Check sheet for the modelled part. Datum: model origin and axes. Units: mm. Round coordinates to 2 decimals unless told otherwise and drop trailing zeros. Write each loop counter-clockwise with the first axis right and the second up, starting at its lowest first coordinate (ties: lowest second). Pieces come first, ordered by that corner, then holes. Notation, with made-up numbers: M 2,36 L 10,36 A12 cw 10,46 Z; hole C -36,-4.75 d6. An arc over 180 degrees is marked long. Answer in a Markdown table with one row per item.
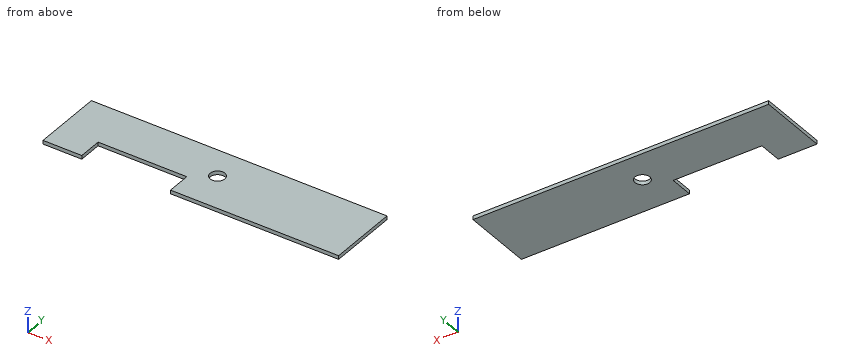
```python
from build123d import *

# Parameters (mm, degrees)
EXTRUDE_1_DEPTH     = 5
SKETCH_2_R          = 10
CUT_EXTRUDE_1_DEPTH = 10


with BuildPart() as part:
    # 草图1 → 凸台-拉伸1 (new body)
    with BuildSketch(Plane.XY):
        Polygon((-255.102040816, 148.567224711), (144.897959184, 148.567224711), (144.897959184, 53.567224711), (92.397959184, 53.567224711), (-27.602040816, 53.567224711), (-82.602040816, 53.567224711), (-82.602040816, 85.567224711), (-202.602040816, 85.567224711), (-202.602040816, 53.567224711), (-255.102040816, 53.567224711), align=None)
    extrude(amount=EXTRUDE_1_DEPTH)

    # 草图2 → 切除-拉伸1 (cut)
    with BuildSketch(Plane.XY.offset(5)):
        with Locations((-55.102040816, 106.067224711)):
            Circle(SKETCH_2_R)
    extrude(amount=-CUT_EXTRUDE_1_DEPTH, mode=Mode.SUBTRACT)


solid = part.part
```
1. Section check B-B, the plane x = -58. Record the cut outline in (y, z), and give its area (3 significant figures).
Found:
| item | result |
|---|---|
| outline | M 53.57,0 L 96.5,0 L 96.5,5 L 53.57,5 Z; M 115.64,0 L 148.57,0 L 148.57,5 L 115.64,5 Z |
| area | 379 mm2 |
2. Section check D-D, the plane x = -114. Record the cut outline in (y, z), and give its area (3 significant figures).
Found:
| item | result |
|---|---|
| outline | M 85.57,0 L 148.57,0 L 148.57,5 L 85.57,5 Z |
| area | 315 mm2 |
3. Scan lines: L1, parallel to X at y = 64.5, z = 2.5; L2, parallel to Y at x = -138.5, z = 0.5; L3, parallel to Y at x = -51.5, z = 3.8. Record each from-to range of solid material in increasing order.
Found:
| item | result |
|---|---|
| L1 | x = -255.1 to -202.6, -82.6 to 144.9 |
| L2 | y = 85.57 to 148.57 |
| L3 | y = 53.57 to 96.74, 115.4 to 148.57 |
4. Section check A-A, the plane y = 61.5. Record the cut outline in (x, z), and give its area (3 significant figures).
Found:
| item | result |
|---|---|
| outline | M -255.1,0 L -202.6,0 L -202.6,5 L -255.1,5 Z; M -82.6,0 L 144.9,0 L 144.9,5 L -82.6,5 Z |
| area | 1,400 mm2 |
5. Go/stop test with flat-tipped pins: pin 1 (16 mm diameter, centred on x = -55.1, y = 106.07, fed in from -Z); pin 2 (2.5 mm diameter, centred on x = -114.5, z = 3, fed in from -Y). Record where each tip stops, or that it passes through.
Found:
| item | result |
|---|---|
| pin 1 | passes through |
| pin 2 | stops at y = 85.57 |
6. Section check C-C, the plane z = 0.8. Record the cut outline in (x, y), and give its area (3 significant figures).
Found:
| item | result |
|---|---|
| outline | M -255.1,53.57 L -202.6,53.57 L -202.6,85.57 L -82.6,85.57 L -82.6,53.57 L 144.9,53.57 L 144.9,148.57 L -255.1,148.57 Z; hole C -55.1,106.07 d20 |
| area | 33,800 mm2 |
